```python
from build123d import *

# Parameters (mm, degrees)
SKETCH_2_W               = 240.549430728
SKETCH_2_H               = 149.540933388
EXTRUDE_1_DEPTH          = 5
SKETCH_6_W               = 93.246571425
SKETCH_6_H               = 149.540933388
EXTRUDE_4_DEPTH          = 5
SKETCH_8_W               = 274.716709757
SKETCH_8_H               = 58.51354913
EXTRUDE_6_DEPTH          = 5
CUT_EXTRUDE_2_DEPTH      = 252.755772101
CUT_EXTRUDE_2_DEPTH_BACK = 252.755772101
SKETCH_9_W               = 59.079292396
SKETCH_9_H               = 149.540933388
SKETCH_10_W              = 104.703380117
SKETCH_10_H              = 208.054482518
CUT_EXTRUDE_3_DEPTH      = 10
SKETCH_12_W              = 200
SKETCH_12_H              = 200
EXTRUDE_7_DEPTH          = 5
SKETCH_13_OUTSIDE_W      = 259.728
SKETCH_13_OUTSIDE_H      = 267.782
SKETCH_13_OUTSIDE_W_2    = 200
SKETCH_13_OUTSIDE_H_2    = 200
CUT_EXTRUDE_4_DEPTH      = 278.64321362
EXTRUDE_START            = -75
SKETCH_18_R              = 5.25
EXTRUDE_9_DEPTH          = 10
EXTRUDE_START_2          = -50
EXTRUDE_10_DEPTH         = 15
EXTRUDE_START_3          = -91.2
EXTRUDE_11_DEPTH         = 15
EXTRUDE_12_REACH         = 286.904
SKETCH_20_R              = 5.25
SKETCH_26_W              = 200
SKETCH_26_H              = 5
EXTRUDE_13_DEPTH         = 100
SKETCH_27_W              = 200
SKETCH_27_H              = 5
CUT_EXTRUDE_5_DEPTH      = 30
EXTRUDE_14_DEPTH         = 10
SKETCH_29_W              = 60
SKETCH_29_H              = 9
EXTRUDE_15_DEPTH         = 10
HOLE_WIZARD_M4_1_D       = 3.3
HOLE_WIZARD_M4_2_D       = 3.3
HOLE_WIZARD_M4_3_D       = 3.3
EXTRUDE_16_DEPTH         = 10
SKETCH_37_W              = 60
SKETCH_37_H              = 9
EXTRUDE_17_DEPTH         = 10
HOLE_WIZARD_M4_4_D       = 3.3
EXTRUDE_START_4          = -3.5
SKETCH_40_R              = 5.25
SKETCH_40_R_2            = 3.25
EXTRUDE_18_DEPTH         = 46.5
CUT_EXTRUDE_START        = -3.5
SKETCH_41_R              = 5.25
SKETCH_41_R_2            = 3.25
CUT_EXTRUDE_6_DEPTH      = 3.5
HOLE_WIZARD_M4_5_D       = 3.3
SKETCH_44_W              = 200
SKETCH_44_H              = 5
CUT_EXTRUDE_7_DEPTH      = 100


with BuildPart() as part:
    # 草图2 → 凸台-拉伸1 (new body)
    with BuildSketch(Plane(origin=(0, 0, 0), x_dir=(1, 0, 0), z_dir=(0, 1, 0))):
        Rectangle(SKETCH_2_W, SKETCH_2_H)
    extrude(amount=EXTRUDE_1_DEPTH)

    # 草图6 → 凸台-拉伸4 (add)
    with BuildSketch(Plane(origin=(0, 5, 0), x_dir=(1, 0, 0), z_dir=(0, 1, 0))):
        with Locations((166.898001077, 0)):
            Rectangle(SKETCH_6_W, SKETCH_6_H)
    extrude(amount=-EXTRUDE_4_DEPTH)

    # 草图8 → 凸台-拉伸6 (add)
    with BuildSketch(Plane(origin=(0, 5, 0), x_dir=(1, 0, 0), z_dir=(0, 1, 0))):
        with Locations((76.162931911, -104.027241259)):
            Rectangle(SKETCH_8_W, SKETCH_8_H)
    extrude(amount=-EXTRUDE_6_DEPTH)

    # 草图9 → 切除-拉伸2 (cut, two sides: drawn at the far end of the back side and taken through both)
    with BuildSketch(Plane(origin=(0, 5, 0), x_dir=(1, 0, 0), z_dir=(0, 1, 0)).offset(-CUT_EXTRUDE_2_DEPTH_BACK)):
        with Locations((-90.735069166, 0)):
            Rectangle(SKETCH_9_W, SKETCH_9_H)
    extrude(amount=CUT_EXTRUDE_2_DEPTH + CUT_EXTRUDE_2_DEPTH_BACK, mode=Mode.SUBTRACT)

    # 草图10 → 切除-拉伸3 (cut)
    with BuildSketch(Plane(origin=(0, 5, 0), x_dir=(1, 0, 0), z_dir=(0, 1, 0))):
        with Locations((-8.84373291, -29.256774565)):
            Rectangle(SKETCH_10_W, SKETCH_10_H)
    extrude(amount=-CUT_EXTRUDE_3_DEPTH, mode=Mode.SUBTRACT)

    # 草图12 → 凸台-拉伸7 (add)
    with BuildSketch(Plane(origin=(0, 5, 0), x_dir=(1, 0, 0), z_dir=(0, 1, 0))):
        with Locations((143.507957149, -25.229533306)):
            Rectangle(SKETCH_12_W, SKETCH_12_H)
    extrude(amount=-EXTRUDE_7_DEPTH)

    # 草图13 outside → 切除-拉伸4 (cut, through all)
    with BuildSketch(Plane(origin=(0, 5, 0), x_dir=(1, 0, 0), z_dir=(0, 1, 0))):
        with Locations((143.508, -29.257)):
            Rectangle(SKETCH_13_OUTSIDE_W, SKETCH_13_OUTSIDE_H)
        with Locations((143.507957149, -25.229533306)):
            Rectangle(SKETCH_13_OUTSIDE_W_2, SKETCH_13_OUTSIDE_H_2, mode=Mode.SUBTRACT)
    extrude(amount=-CUT_EXTRUDE_4_DEPTH, mode=Mode.SUBTRACT)

    # 草图18 → 凸台-拉伸9 (add)
    with BuildSketch(Plane.XY.offset(125.229533306).offset(EXTRUDE_START)):
        with BuildLine():
            Line((95.507957149, 14), (95.507957149, 75))
            ThreePointArc((95.507957149, 75), (88.507957149, 82), (81.507957149, 75))
            Line((81.507957149, 75), (81.507957149, 14))
            Line((81.507957149, 14), (68.507957149, 14))
            Line((68.507957149, 14), (68.507957149, 5))
            Line((68.507957149, 5), (108.507957149, 5))
            Line((108.507957149, 5), (108.507957149, 14))
            Line((108.507957149, 14), (95.507957149, 14))
        make_face()
        with Locations((88.507957149, 75)):
            Circle(SKETCH_18_R, mode=Mode.SUBTRACT)
    extrude_9 = extrude(amount=-EXTRUDE_9_DEPTH)

    # 镜向1: 凸台-拉伸9 across plane
    add(extrude_9.mirror(Plane.XY.offset(25.229533306)))

    # 草图16 → 凸台-拉伸10 (add)
    with BuildSketch(Plane(origin=(243.507957149, 0, 0), x_dir=(0, 0, -1), z_dir=(1, 0, 0)).offset(EXTRUDE_START_2)):
        with BuildLine():
            Line((-53.779533306, 14), (-53.779533306, 93))
            Line((-53.779533306, 93), (-67.779533306, 93))
            Line((-67.779533306, 93), (-67.779533306, 87.085631965))
            ThreePointArc((-67.779533306, 87.085631965), (-69.779533306, 62.75), (-71.779533306, 87.085631965))
            Line((-71.779533306, 87.085631965), (-71.779533306, 93))
            Line((-71.779533306, 93), (-85.779533306, 93))
            Line((-85.779533306, 93), (-85.779533306, 14))
            Line((-85.779533306, 14), (-99.779533306, 14))
            Line((-99.779533306, 14), (-99.779533306, 5))
            Line((-99.779533306, 5), (-39.779533306, 5))
            Line((-39.779533306, 5), (-39.779533306, 14))
            Line((-39.779533306, 14), (-53.779533306, 14))
        make_face()
    extrude(amount=-EXTRUDE_10_DEPTH)

    # 草图19 → 凸台-拉伸11 (add)
    with BuildSketch(Plane(origin=(243.507957149, 0, 0), x_dir=(0, 0, -1), z_dir=(1, 0, 0)).offset(EXTRUDE_START_3)):
        with BuildLine():
            Line((37.990466694, 14), (37.990466694, 92.933566106))
            Line((37.990466694, 92.933566106), (23.990466694, 92.933566106))
            Line((23.990466694, 92.933566106), (23.990466694, 86.933566106))
            ThreePointArc((23.990466694, 86.933566106), (21.990466694, 62.9), (19.990466694, 86.933566106))
            Line((19.990466694, 86.933566106), (19.990466694, 92.933566106))
            Line((19.990466694, 92.933566106), (5.990466694, 92.933566106))
            Line((5.990466694, 92.933566106), (5.990466694, 14))
            Line((5.990466694, 14), (-8.009533306, 14))
            Line((-8.009533306, 14), (-8.009533306, 5))
            Line((-8.009533306, 5), (51.990466694, 5))
            Line((51.990466694, 5), (51.990466694, 14))
            Line((51.990466694, 14), (37.990466694, 14))
        make_face()
    extrude(amount=-EXTRUDE_11_DEPTH)

    # 草图20 → 凸台-拉伸12 (add, up to next)
    with BuildSketch(Plane(origin=(0, 0, 40.229533306), x_dir=(-1, 0, 0), z_dir=(0, 0, -1)), mode=Mode.PRIVATE) as extrude_12_sk1:
        with BuildLine():
            Line((-108.507957149, 5), (-68.507957149, 5))
            Line((-68.507957149, 5), (-68.507957149, 14))
            Line((-68.507957149, 14), (-81.507957149, 14))
            Line((-81.507957149, 14), (-81.507957149, 75))
            ThreePointArc((-81.507957149, 75), (-88.507957149, 82), (-95.507957149, 75))
            Line((-95.507957149, 75), (-95.507957149, 14))
            Line((-95.507957149, 14), (-108.507957149, 14))
            Line((-108.507957149, 14), (-108.507957149, 5))
        make_face()
        with Locations(Location((-88.507957149, 75, 0), (0, 0, 180))):
            Circle(SKETCH_20_R, mode=Mode.SUBTRACT)
    extrude_12_tool1 = extrude(extrude_12_sk1.sketch, amount=EXTRUDE_12_REACH, mode=Mode.PRIVATE) - part.part
    add(extrude_12_tool1.solids().sort_by_distance((88.507957, 33.984391, 40.229533))[0])

    # 草图26 → 凸台-拉伸13 (add)
    with BuildSketch(Plane(origin=(243.507957149, 0, 0), x_dir=(0, 0, -1), z_dir=(1, 0, 0))):
        with Locations((-25.229533306, 2.5)):
            Rectangle(SKETCH_26_W, SKETCH_26_H)
    extrude(amount=EXTRUDE_13_DEPTH)

    # 草图27 → 切除-拉伸5 (cut)
    with BuildSketch(Plane(origin=(343.507957149, 0, 0), x_dir=(0, 0, -1), z_dir=(1, 0, 0))):
        with Locations((-25.229533306, 2.5)):
            Rectangle(SKETCH_27_W, SKETCH_27_H)
    extrude(amount=-CUT_EXTRUDE_5_DEPTH, mode=Mode.SUBTRACT)

    # 草图28 → 凸台-拉伸14 (add)
    with BuildSketch(Plane(origin=(193.507957149, 0, 0), x_dir=(0, 0, -1), z_dir=(1, 0, 0))):
        Polygon((-85.779533306, 14), (-53.779533306, 14), (-39.779533306, 14), (-39.779533306, 5), (-99.779533306, 5), (-99.779533306, 14), align=None)
    extrude(amount=EXTRUDE_14_DEPTH)

    # 草图29 → 凸台-拉伸15 (add)
    with BuildSketch(Plane.ZY.offset(-178.507957149)):
        with Locations((69.779533306, 9.5)):
            Rectangle(SKETCH_29_W, SKETCH_29_H)
    extrude(amount=EXTRUDE_15_DEPTH)

    # M4 螺纹孔1 (through all)
    with Locations(Plane(origin=(0, 14, 0), x_dir=(1, 0, 0), z_dir=(0, 1, 0))):
        with Locations((174.507957149, -47.779533306), (197.507957149, -47.779533306), (197.507957149, -91.779533306), (174.507957149, -91.779533306)):
            Hole(HOLE_WIZARD_M4_1_D / 2)

    # M4 螺纹孔2 (through all)
    with Locations(Plane.XY.offset(85.779533306)):
        with Locations((186.007957149, 89)):
            Hole(HOLE_WIZARD_M4_2_D / 2)

    # M4 螺纹孔3 (through all)
    with Locations(Plane.XY.offset(-5.990466694)):
        with Locations((144.807957149, 88.933566106)):
            Hole(HOLE_WIZARD_M4_3_D / 2)

    # 草图36 → 凸台-拉伸16 (add)
    with BuildSketch(Plane(origin=(152.307957149, 0, 0), x_dir=(0, 0, -1), z_dir=(1, 0, 0))):
        Polygon((5.990466694, 14), (37.990466694, 14), (51.990466694, 14), (51.990466694, 5), (-8.009533306, 5), (-8.009533306, 14), align=None)
    extrude(amount=EXTRUDE_16_DEPTH)

    # 草图37 → 凸台-拉伸17 (add)
    with BuildSketch(Plane.ZY.offset(-137.307957149)):
        with Locations((-21.990466694, 9.5)):
            Rectangle(SKETCH_37_W, SKETCH_37_H)
    extrude(amount=EXTRUDE_17_DEPTH)

    # M4 螺纹孔4 (through all)
    with Locations(Plane(origin=(0, 14, 0), x_dir=(1, 0, 0), z_dir=(0, 1, 0))):
        with Locations((133.307957149, 43.990466694), (156.307957149, 43.990466694), (156.307957149, -0.009533306), (133.307957149, -0.009533306)):
            Hole(HOLE_WIZARD_M4_4_D / 2)

    # 草图40 → 凸台-拉伸18 (add)
    with BuildSketch(Plane.XY.offset(50.229533306).offset(EXTRUDE_START_4)):
        with Locations((88.507957149, 75)):
            Circle(SKETCH_40_R)
        with Locations((88.507957149, 75)):
            Circle(SKETCH_40_R_2, mode=Mode.SUBTRACT)
    extrude(amount=-EXTRUDE_18_DEPTH)

    # 草图41 → 切除-拉伸6 (cut)
    with BuildSketch(Plane(origin=(0, 0, 0.229533306), x_dir=(-1, 0, 0), z_dir=(0, 0, -1)).offset(CUT_EXTRUDE_START)):
        with Locations(Location((-88.507957149, 75, 0), (0, 0, 180))):
            Circle(SKETCH_41_R)
        with Locations(Location((-88.507957149, 75, 0), (0, 0, 180))):
            Circle(SKETCH_41_R_2, mode=Mode.SUBTRACT)
    extrude(amount=CUT_EXTRUDE_6_DEPTH, mode=Mode.SUBTRACT)

    # M4 螺纹孔5 (through all)
    with Locations(Plane(origin=(0, 14, 0), x_dir=(1, 0, 0), z_dir=(0, 1, 0))):
        with Locations((73.507957149, -8.229533306), (103.507957149, -8.229533306), (103.507957149, -42.229533306), (73.507957149, -42.229533306)):
            Hole(HOLE_WIZARD_M4_5_D / 2)

    # 草图44 → 切除-拉伸7 (cut)
    with BuildSketch(Plane(origin=(313.507957149, 0, 0), x_dir=(0, 0, -1), z_dir=(1, 0, 0))):
        with Locations((-25.229533306, 2.5)):
            Rectangle(SKETCH_44_W, SKETCH_44_H)
    extrude(amount=-CUT_EXTRUDE_7_DEPTH, mode=Mode.SUBTRACT)


solid = part.part
```
Geometry: final body of the model. Coordinates: model frame, mm. A direction names the side the tool comes from. Round coordinates to 2 decimals unless told otherwise and drop trailing zeros. Loops run counter-clockwise (first coordinate to the right, second up) from the corner with the lowest first, then second, coordinate; pieces in that order, holes last. Notation, with made-up numbers: (66.25, 74) -> (94.25, 74) arc R30 ccw to (94.25, 105) -> close; hole circle Ø4 at (-21, 81). An arc over 180 degrees is marked (long way). Use one line per item in the form item = value. Start each with the question number.
1) Section C-C on z = 111. Output: boundary loops of the cut face in (x, y), then the cut area to 3 significant figures.
2) Access query for faces 1 (the flat face through (186, 91, 71.78)), 2 (the flat face through (145, 54, -5.99)), 3 (the flat face through (81.508, 45, 26)), 4 (the flat face through (102, 14, 26)). Directions: +Z, -Z, +X, -X, +Y, -Y. A direction counts if a zero-diameter tool reaches every point of the face in a straight line with its end or side. Return the directions, or none.
3) Section B-B on x = 190. Output: boundary loops of the cut face in (y, z).
4) Line query: L1, parallel to X at y = 75, z = 34; L2, parallel to Z at x = 143, y = 75; L3, parallel to Y at x = 93, z = 64.5. Output: solid intervals per line, ascending.
5) First-contact query: P1, Ø4, axis at x = 156.31, z = -43.99, coming from the +Y side; P2, Ø4.5, axis at x = 182, y = 10.5, coming from the +Z side; P3, Ø4, axis at y = 26, z = -36.5, coming from the +X side; P4, Ø2, axis at x = 197.51, z = 47.78, coming from the -Y side. Flat tips, straight axial feed; report the tip coordinate or a pass-through.
6) Draft query along X for faces 5 (the flat face through (127, 2, 125.23)), 6 (the flat face through (152.308, 45, -22)), 7 (the flat face through (88.4, 71.6, 46.73)), 8 (the flat face through (108.508, 10, 26)). Return one class per face: released by +X, released by -X, zero draft, split by the parting line, or undercut.
7) Section D-D on x = 125. Output: boundary loops of the cut face in (y, z).
8) Section A-A on y = 20. Output: boundary loops of the cut face in (x, z), then the cut area to 3 significant figures.
Response:
q1.outline = (43.51, 0) -> (213.51, 0) -> (213.51, 5) -> (43.51, 5) -> close
q1.area = 850 mm^2
q2.face_1 = +X, -X, +Y
q2.face_2 = +Z, +X, -X, +Y
q2.face_3 = +Z, -Z, -X, +Y
q2.face_4 = +Z, -Z, +X, +Y
q3.outline = (0, -74.77) -> (5, -74.77) -> (5, 39.78) -> (14, 39.78) -> (14, 53.78) -> (93, 53.78) -> (93, 67.78) -> (87.09, 67.78) arc R12.25 cw (long way) to (87.09, 71.78) -> (93, 71.78) -> (93, 85.78) -> (14, 85.78) -> (14, 99.78) -> (5, 99.78) -> (5, 125.23) -> (0, 125.23) -> close
q4.L1 = 81.51 to 85.26, 91.76 to 95.51
q4.L2 = -37.99 to -34.09, -9.89 to -5.99
q4.L3 = 0 to 5
q5.P1 = 14
q5.P2 = 99.78
q5.P3 = 152.31
q5.P4 = through
q6.face_5 = zero draft
q6.face_6 = released by +X
q6.face_7 = undercut
q6.face_8 = undercut
q7.outline = (0, -74.77) -> (5, -74.77) -> (5, 125.23) -> (0, 125.23) -> close
q8.outline = (81.51, 0.23) -> (95.51, 0.23) -> (95.51, 50.23) -> (81.51, 50.23) -> close; (137.31, -37.99) -> (152.31, -37.99) -> (152.31, -5.99) -> (137.31, -5.99) -> close; (178.51, 53.78) -> (193.51, 53.78) -> (193.51, 85.78) -> (178.51, 85.78) -> close
q8.area = 1,660 mm^2
